from build123d import *


with BuildPart() as part:
    # Sweep1: sweep along a curve in space
    with BuildLine() as sweep1_path:
        Line((409.121226164, 1758.017106037, 1349.85455637), (409.121226164, 1783.417106037, 1146.65455637))
        Line((409.121226164, 1758.017106037, 1349.85455637), (409.121226164, 1758.017106037, 1553.05455637))
        Line((409.121226164, 1758.017106037, 1553.05455637), (409.121226164, 1783.417106037, 1764.897256503))
    # 3DSketch2 → Sweep1 (sweep)
    with BuildSketch(Plane(origin=(396.244700962, 1770.717106037, 1146.65455637), x_dir=(0.7119701649816974, 0.7022097152389267, -7.366387974552788e-14), z_dir=(0, 0, -1))):
        Polygon((0, 0), (18.335403545, 18.084042191), (36.171530312, 0), (17.836126767, -18.084042191), align=None)
    sweep(path=sweep1_path.line, transition=Transition.RIGHT)


solid = part.part
Read the model definition and answer for the solid it produces. Units are mm, in the model's axes. A direction names the side the tool comes from. Round coordinates to 2 decimals unless told otherwise and drop trailing zeros. Loops run counter-clockwise (first coordinate to the right, second up) from the corner with the lowest first, then second, coordinate; pieces in that order, holes last. Notation, with made-up numbers: (82.25, 33) - (127.25, 33) arc R17 ccw to (127.25, 45) - close; hole circle Ø2 at (18, 86.25). An arc over 180 degrees is marked (long way). One line per question, with ' | ' between items. Start each with the question number.
Q1. Find the intervals of material crossed by L1, parallel to Y at x = 408.25, z = 1539; L2, parallel to Y at x = 419, z = 1721, in increasing order.
Q2. Section C-C on y = 1764 is taken. Give the vertices of the cut face in (x, z), plus the area to 3 significant figures.
Q3. Section D-D on z = 1433.5 is taken. Give the vertices of the cut face in (x, y).
Q4. Section A-A on y = 1786 is taken. Give the vertices of the cut face in (x, z).
Q5. Section B-B on x = 401.5 is taken. Give the vertices of the cut face in (y, z).
Q6. For faces 4 (the flat face through (408.941, 1783.59, 1764.854)), 5 (the flat face through (408.941, 1783.547, 1247.219)), determine the directions among +Z, -Z, +X, -X, +Y, -Y from which every point of the face is accessible in a straight line to the end or side of a thin tool.
Q7. Flat-ended cylindrical pins translate along their axes: pin 1 (1.5 mm diameter, centred on x = 399.5, z = 1273.5, fed in from +Y); pin 2 (6 mm diameter, centred on x = 404.5, z = 1464.5, fed in from +Y); pin 3 (10 mm diameter, centred on y = 1777, z = 1494, fed in from +X); pin 4 (6 mm diameter, centred on x = 408, z = 1303.5, fed in from +Y). Find the tip coordinate at first contact, or state that the pin passes through.
Q8. For a pull along Z with two mould halves and no side action, classify faces 1 (the flat face through (408.941, 1783.005, 1655.601)), 2 (the flat face through (409, 1784, 1146.655)), 3 (the flat face through (409, 1745.415, 1450)) as +Z half, -Z half, draft (parallel to the pull), parting line (faces both ways), or undercut.
Established:
1) L1: 1745.42 to 1770.62 | L2: 1765.46 to 1790.85
2) outline: (396.24, 1200.39) - (422, 1200.39) - (422, 1708.81) - (396.24, 1708.81) - close | area: 13,100 mm²
3) outline: (396.24, 1745.42) - (422, 1745.42) - (422, 1770.62) - (396.24, 1770.62) - close
4) outline: (396.24, 1146.65) - (422, 1146.65) - (422, 1227.59) - (396.24, 1227.59) - close; (396.24, 1680.58) - (422, 1680.58) - (422, 1764.26) - (396.24, 1764.26) - close
5) outline: (1745.42, 1349.07) - (1770.72, 1146.65) - (1796.12, 1146.65) - (1770.62, 1350.64) - (1770.62, 1552.3) - (1795.74, 1761.83) - (1771.09, 1767.96) - (1745.42, 1553.81) - close
6) face 4: +Z, +X, -X, +Y | face 5: +X, -X, +Y
7) pin 1: y = 1780.36 | pin 2: y = 1770.62 | pin 3: through | pin 4: y = 1776.89
8) face 1: undercut | face 2: -Z half | face 3: draft
